Drawing for the job (mm, zero at the part's lowest x, y, z). A direction names the side the tool comes from. Give positions to 0.01 mm unless a question says otherwise; leave off trailing zeros. Order: outer loops, then holes, each group sorted by start corner. A loop starts at its lowest first (then second) coordinate and runs counter-clockwise, first axis right, second up. Notation, with made-up numbers: (-25.75, 0.25) -> (12.25, 0.25) arc R17 ccw to (12.25, 24.25) -> close; hole circle Ø10 at (9, -13). An arc over 180 degrees is marked (long way). Use one line per item in the form item = value. Start each with the question number.
1) Drop flat-ended pins along their axis: P1, Ø3.5, axis at x = 20, z = 15, coming from the +Y side; P2, Ø1, axis at x = 5, y = 5, coming from the +Z side; P3, Ø1.9, axis at x = 38.5, y = 4.5, coming from the -Z side; P4, Ø1.9, axis at y = 4.5, z = 26, coming from the +X side. Give the stop position or say it passes through.
2) Probe line 1 (X direction, y = 2, z = 26.75); line 2 (X direction, y = 3.25, z = 15) (3 decimals); line 3 (Z direction, x = 20, y = 4) (3 decimals). List the from-to ranges inside material, lowest first.
3) Tool access for the marked faces 5, 6, 7, 8 and 9: list every direction of +Z, -Z, +X, -X, +Y, -Y with a clear straight run to the whole face (end or side of a thin tool).
4) Cut at D-D, the plane x = 35.5. Give the cut face in (y, z), and give its area (3 significant figures).
5) Mould opens along Z. For the marked faces 1, 2, 3 and 4 say: pulls with the +Z half, pulls with the -Z half, needs draft (parallel to the pull), parting line crosses it, or undercut.
6) Cut at B-B, the plane y = 4.75. Give the cut face in (x, z) (3 decimals), and give its area (3 significant figures).
7) Cut at A-A, the plane z = 26. Give the cut face in (x, y).
8) Cut at C-C, the plane z = 8. Give the cut face in (x, y), and give its area (3 significant figures).
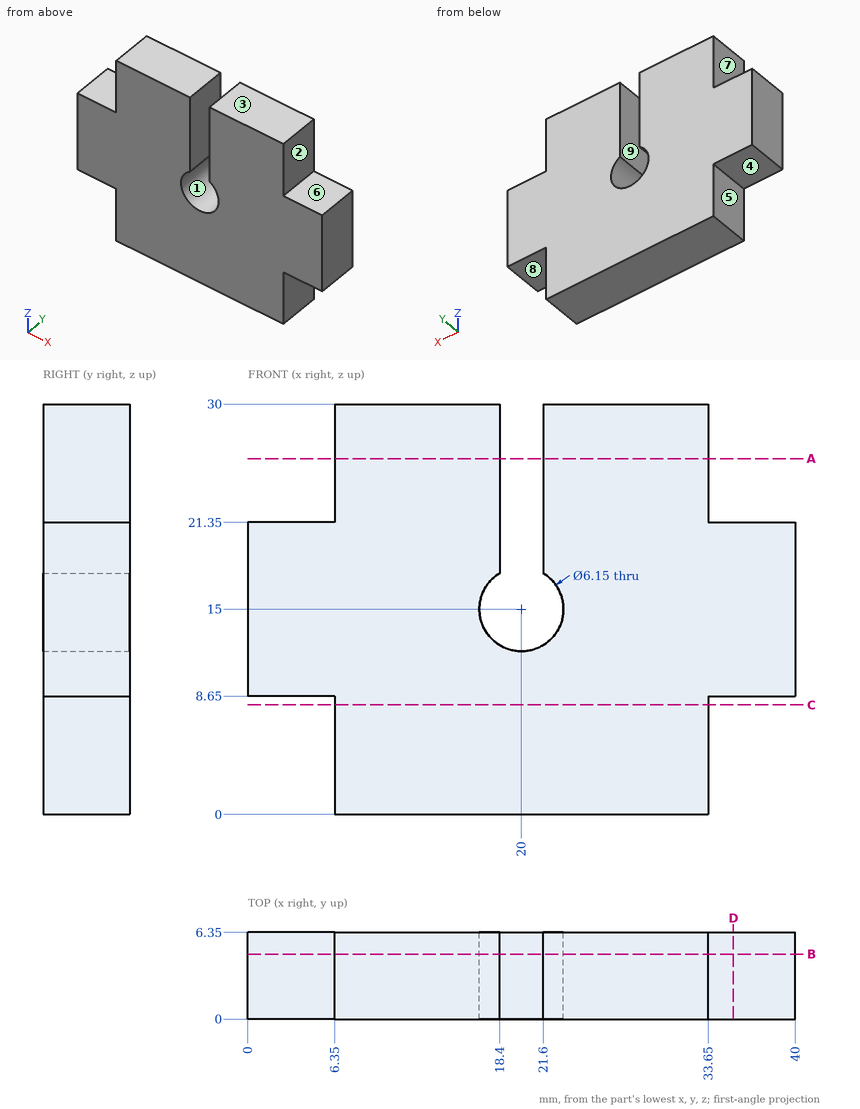
Result:
q1.P1 = through
q1.P2 = 21.35
q1.P3 = 8.65
q1.P4 = 33.65
q2.line_1 = 6.35 to 18.4, 21.6 to 33.65
q2.line_2 = 0 to 16.925, 23.075 to 40
q2.line_3 = 0 to 11.925
q3.face_5 = -Z, -X, +Y, -Y
q3.face_6 = +Z, +X, +Y, -Y
q3.face_7 = +Z, -X, +Y, -Y
q3.face_8 = -Z, +X, +Y, -Y
q3.face_9 = +Z, +Y, -Y
q4.outline = (0, 8.65) -> (6.35, 8.65) -> (6.35, 21.35) -> (0, 21.35) -> close
q4.area = 80.6 mm²
q5.face_1 = undercut
q5.face_2 = needs draft
q5.face_3 = pulls with the +Z half
q5.face_4 = pulls with the -Z half
q6.outline = (0, 8.65) -> (6.35, 8.65) -> (6.35, 0) -> (33.65, 0) -> (33.65, 8.65) -> (40, 8.65) -> (40, 21.35) -> (33.65, 21.35) -> (33.65, 30) -> (21.6, 30) -> (21.6, 17.626) arc R3.075 cw (long way) to (18.4, 17.626) -> (18.4, 30) -> (6.35, 30) -> (6.35, 21.35) -> (0, 21.35) -> close
q6.area = 912 mm²
q7.outline = (6.35, 0) -> (18.4, 0) -> (18.4, 6.35) -> (6.35, 6.35) -> close; (21.6, 0) -> (33.65, 0) -> (33.65, 6.35) -> (21.6, 6.35) -> close
q8.outline = (6.35, 0) -> (33.65, 0) -> (33.65, 6.35) -> (6.35, 6.35) -> close
q8.area = 173 mm²
